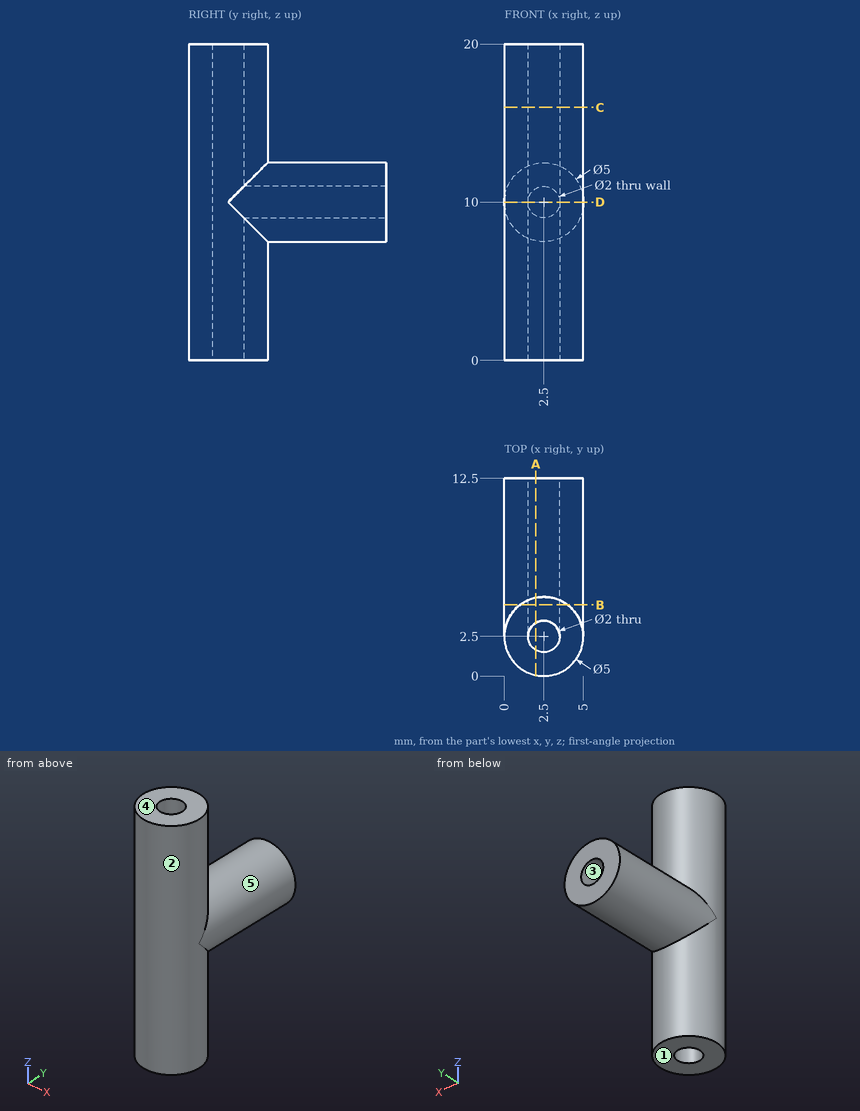
Can you work these out from the drawing? Everything is in mm from the part's minimum corner. A direction names the side the tool comes from. Give positions to 0.01 mm unless a question says otherwise; leave off trailing zeros. Loops run counter-clockwise (first coordinate to the right, second up) from the corner with the lowest first, then second, coordinate; pieces in that order, holes last. Notation, with made-up numbers: (-20, 55) -> (25, 55) arc R15 ccw to (25, 61) -> close; hole circle Ø6 at (10, 29.25). An arc over 180 degrees is marked (long way). Return JSON: item names as keys, results as strings.
Item 1: If we section it at C-C on z = 16: List the corners of the cut face in (x, y) for me, plus the area to 3 significant figures.
Geometry results:
{"outline": "circle Ø5 at (2.5, 2.5); hole circle Ø2 at (2.5, 2.5)", "area": "16.5 mm²"}
Item 2: We'd pull the mould along Z, two halves only. Please class the marked faces 1, 2 and 3: +Z half, -Z half, draft (parallel to the pull), parting line (faces both ways), or undercut.
Geometry results:
{"face 1": "-Z half", "face 2": "draft", "face 3": "undercut"}
Item 3: If we section it at A-A on x = 2: List the corners of the cut face in (y, z) for me, plus the area to 3 significant figures.
Geometry results:
{"outline": "(0.05, 0) -> (1.63, 0) -> (1.63, 20) -> (0.05, 20) -> close; (3.37, 0) -> (4.95, 0) -> (4.95, 7.55) -> (12.5, 7.55) -> (12.5, 9.13) -> (3.37, 9.13) -> close; (3.37, 10.87) -> (12.5, 10.87) -> (12.5, 12.45) -> (4.95, 12.45) -> (4.95, 20) -> (3.37, 20) -> close", "area": "84.5 mm²"}
Item 4: If we section it at B-B on y = 4.5: List the corners of the cut face in (x, z) for me.
Geometry results:
{"outline": "(1, 0) -> (4, 0) -> (4, 8) arc R2.5 ccw to (4, 12) -> (4, 20) -> (1, 20) -> (1, 12) arc R2.5 ccw to (1, 8) -> close; hole circle Ø2 at (2.5, 10)"}
Item 5: If we section it at D-D on z = 10: List the corners of the cut face in (x, y) for me, plus the area to 3 significant figures.
Geometry results:
{"outline": "(0, 2.5) arc R2.5 ccw to (5, 2.5) -> (5, 12.5) -> (3.5, 12.5) -> (3.5, 2.5) arc R1 cw to (1.5, 2.5) -> (1.5, 12.5) -> (0, 12.5) -> close", "area": "38.2 mm²"}
Item 6: I need wall thicknesses on L1, parallel to X at y = 5.5, z = 10; L2, parallel to Y at x = 2.5, z = 10.25. Which ranges of each line are inside material? Lowest first, please. Write a range as from..to.
Geometry results:
{"L1": "x = 0..1.5, 3.5..5", "L2": "y = 0..1.5"}
Item 7: Which directions (+Z, -Z, +X, -X, +Y, -Y) give clear straight access to the entire face, cutting with the end or side of a thin tool? Please do the marked faces 4 and 5.
Geometry results:
{"face 4": "+Z, +X, -X, +Y, -Y", "face 5": "+Y"}
Item 8: I'm going to push flat-ended pins straight in: pin 1 (1 mm diameter, centred on y = 8, z = 14.5, fed in from -X); pin 2 (2 mm diameter, centred on y = 4.5, z = 6.5, fed in from +X); pin 3 (5 mm diameter, centred on y = 8.5, z = 6, fed in from +X). Where does each tip first touch, or does it pass through?
Geometry results:
{"pin 1": "passes through", "pin 2": "stops at x = 4.79", "pin 3": "stops at x = 4.5"}
